Input: dimensioned drawing with shaded views. Units: mm. Origin: part minimum x, y, z. Round coordinates to 2 decimals unless told otherwise and drop trailing zeros. Loops run counter-clockwise (first coordinate to the right, second up) from the corner with the lowest first, then second, coordinate; pieces in that order, holes last. Notation, with made-up numbers: (49, 71) -> (86, 71) arc R31 cw to (86, 105) -> close; hole circle Ø4 at (74, -13.75). An arc over 180 degrees is marked (long way). Answer as a JSON object with one key per item and string values.
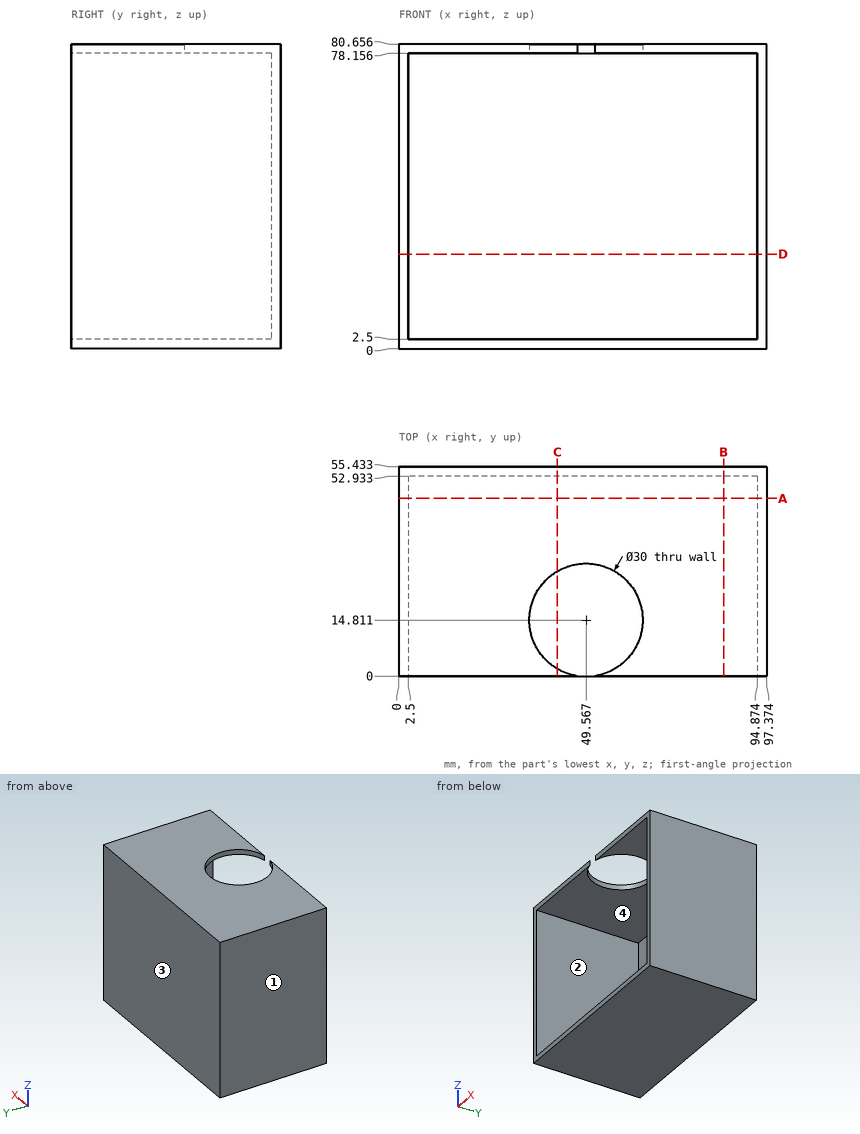
1) Contact query for a flat-ended pin moving along its axis: P1, Ø3, axis at x = 47, y = 7.5, coming from the +Z side. Output: stop coordinate, or through.
Output:
{"P1": "stops at z = 2.5"}
2) Section D-D, the plane z = 25. Output: boundary loops of the cut face in (x, y) (1 decimal).
Output:
{"outline": "(0, 0) -> (2.5, 0) -> (2.5, 52.9) -> (94.9, 52.9) -> (94.9, 0) -> (97.4, 0) -> (97.4, 55.4) -> (0, 55.4) -> close"}
3) Section C-C, the plane x = 42. Output: boundary loops of the cut face in (y, z).
Output:
{"outline": "(0, 0) -> (55.43, 0) -> (55.43, 80.66) -> (27.76, 80.66) -> (27.76, 78.16) -> (52.93, 78.16) -> (52.93, 2.5) -> (0, 2.5) -> close; (0, 78.16) -> (1.86, 78.16) -> (1.86, 80.66) -> (0, 80.66) -> close"}
4) Section B-B, the plane x = 86. Output: boundary loops of the cut face in (y, z).
Output:
{"outline": "(0, 0) -> (55.43, 0) -> (55.43, 80.66) -> (0, 80.66) -> (0, 78.16) -> (52.93, 78.16) -> (52.93, 2.5) -> (0, 2.5) -> close"}
5) Ray query, probe 1 along Z at (x, y) = (65, 23); probe 2 along X at (y, z) = (22, 53.5) (1 decimal); probe 3 along Y at (x, z) = (57, 59.5). Return the intervals inside material, ascending.
Output:
{"probe 1": "z = 0 to 2.5, 78.16 to 80.66", "probe 2": "x = 0 to 2.5, 94.9 to 97.4", "probe 3": "y = 52.93 to 55.43"}
6) Section A-A, the plane y = 47. Output: boundary loops of the cut face in (x, z) (1 decimal).
Output:
{"outline": "(0, 0) -> (97.4, 0) -> (97.4, 80.7) -> (0, 80.7) -> close; hole (2.5, 2.5) -> (94.9, 2.5) -> (94.9, 78.2) -> (2.5, 78.2) -> close"}
7) Draft query along X for the marked faces 1, 2, 3 and 4. Return one class per face: +X half, -X half, draft (parallel to the pull), parting line (faces both ways), or undercut.
Output:
{"face 1": "-X half", "face 2": "undercut", "face 3": "draft", "face 4": "undercut"}
